Read the model definition and answer for the solid it produces. Units are mm, in the model's axes. Face numbers are marked on the shaded views. A direction names the side the tool comes from. Give positions to 0.01 mm unless a question says otherwise; leave off trailing zeros. Order: outer loops, then holes, each group sorted by start corner. A loop starts at its lowest first (then second) coordinate and runs counter-clockwise, first axis right, second up. Notation, with made-up numbers: (-5, 42) - (24, 42) arc R13 ccw to (24, 64) - close; hole circle Ø6 at (85, 55). An arc over 180 degrees is marked (long way). Use a Markdown table: item, result. Add a question column.
1. A cutting plane is placed at C-C on x = 73. Determine the outline of the cut face in (y, z).
2. Which of the six approach directions +Z, -Z, +X, -X, +Y, -Y give full straight-line access (tool end or side, diameter ignored) to the marked faces 1 and 2?
3. A cutting plane is placed at D-D on z = 5. Determine the outline of the cut face in (x, y).
4. A cutting plane is placed at A-A on x = 7. Determine the outline of the cut face in (y, z), and give its area (3 significant figures).
5. A cutting plane is placed at B-B on y = 0. Determine the outline of the cut face in (x, z).
6. Consider L1, parallel to Z at x = 16.5, y = 0; L2, parallel to X at y = -3.75, z = -4.25; L3, parallel to X at y = -0.5, z = -2.75. Determine where each line is inside the solid, lowest interval first.
7. Flat-ended cylindrical pins translate along their axes: P1, Ø3, axis at x = 56, z = -2, coming from the +Y side; P2, Ø2, axis at y = 4.5, z = -4, coming from the +X side. Find the tip coordinate at first contact, or state that the pin passes through.
```python
from build123d import *

# Parameters (mm, degrees)
F0_R     = 4
F0_R_2   = 3
F1_DEPTH = 85
F2_DEPTH = 25
F3_START = 85
F3_DEPTH = 15


# Not quite as in the source:
# - a feature names something its author has since deleted; it is built from what else it names


with BuildPart() as f1:
    # F0 (on Right) → F1 (new body)
    with BuildSketch(Plane.YZ):
        Polygon((-3.7528207105, 6.4999746191), (-7.5055534993, -5.07616e-05), (-3.7527327888, -6.5000253806), (3.7528207105, -6.4999746191), (7.5055534993, 5.07616e-05), (3.7527327888, 6.5000253806), align=None)
        Circle(F0_R, mode=Mode.SUBTRACT)
        Circle(F0_R)
        Circle(F0_R_2, mode=Mode.SUBTRACT)
        Circle(F0_R_2)
    extrude(amount=F1_DEPTH)

    # F0 (on Right) → F2 (cut)
    with BuildSketch(Plane.YZ):
        Circle(F0_R_2)
    extrude(amount=F2_DEPTH, mode=Mode.SUBTRACT)

    # F0 (on Right) → F3 (join)
    with BuildSketch(Plane.YZ.offset(F3_START)):
        Circle(F0_R)
        Circle(F0_R_2, mode=Mode.SUBTRACT)
        Circle(F0_R_2)
    extrude(amount=F3_DEPTH)


solid = f1.part
```
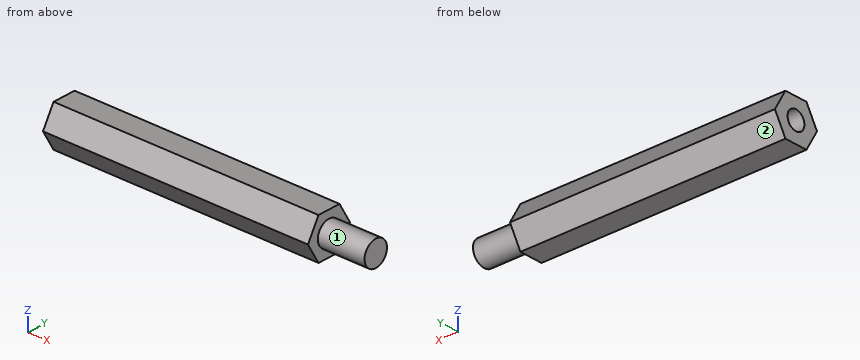
Output values:
| question | item | result |
|---|---|---|
| 1 | outline | (-7.51, 0) - (-3.75, -6.5) - (3.75, -6.5) - (7.51, 0) - (3.75, 6.5) - (-3.75, 6.5) - close |
| 2 | face 1 | +X |
| 2 | face 2 | -Z, +X, -X, +Y |
| 3 | outline | (0, -4.62) - (85, -4.62) - (85, 4.62) - (0, 4.62) - close |
| 4 | outline | (-7.51, 0) - (-3.75, -6.5) - (3.75, -6.5) - (7.51, 0) - (3.75, 6.5) - (-3.75, 6.5) - close; hole circle Ø6 at (0, 0) |
| 4 | area | 118 mm² |
| 5 | outline | (0, -6.5) - (85, -6.5) - (85, -4) - (100, -4) - (100, 4) - (85, 4) - (85, 6.5) - (0, 6.5) - (0, 3) - (25, 3) - (25, -3) - (0, -3) - close |
| 6 | L1 | -6.5 to -3, 3 to 6.5 |
| 6 | L2 | 0 to 85 |
| 6 | L3 | 25 to 100 |
| 7 | P1 | y = 7.22 |
| 7 | P2 | x = 85 |
